```python
from build123d import *

# Parameters (mm, degrees)
SKETCH1_W           = 28.7
SKETCH1_H           = 30.1
BOSS_EXTRUDE1_DEPTH = 10.3
SKETCH2_W           = 22
SKETCH2_H           = 20.1
SKETCH2_R           = 0.95
BOSS_EXTRUDE2_DEPTH = 4
SKETCH4_R           = 0.95
CUT_EXTRUDE1_DEPTH  = 44.979427009


with BuildPart() as part:
    # Sketch1 → Boss-Extrude1 (new body)
    with BuildSketch(Plane.XY):
        with Locations((14.35, 15.05)):
            Rectangle(SKETCH1_W, SKETCH1_H)
    extrude(amount=BOSS_EXTRUDE1_DEPTH)

    # Sketch2 → Boss-Extrude2 (add)
    with BuildSketch(Plane.XY.offset(10.3)):
        with Locations((14.35, 15.05)):
            Rectangle(SKETCH2_W, SKETCH2_H)
        with Locations((6.967324962, 8.304919624)):
            Circle(SKETCH2_R, mode=Mode.SUBTRACT)
        with Locations(Location((6.967324962, 21.795080376, 0), (0, 0, 180))):
            Circle(SKETCH2_R, mode=Mode.SUBTRACT)
        with Locations(Location((21.732675038, 8.304919624, 0), (0, 0, 180))):
            Circle(SKETCH2_R, mode=Mode.SUBTRACT)
        with Locations((21.732675038, 21.795080376)):
            Circle(SKETCH2_R, mode=Mode.SUBTRACT)
    extrude(amount=BOSS_EXTRUDE2_DEPTH)

    # Sketch4 → Cut-Extrude1 (cut, through all)
    with BuildSketch(Plane(origin=(0, 0, 0), x_dir=(-1, 0, 0), z_dir=(0, 0, -1))):
        with Locations((-21.732675038, 21.795080376)):
            Circle(SKETCH4_R)
        with Locations((-21.732675038, 8.304919624)):
            Circle(SKETCH4_R)
        with Locations((-6.967324962, 8.304919624)):
            Circle(SKETCH4_R)
        with Locations((-6.967324962, 21.795080376)):
            Circle(SKETCH4_R)
    extrude(amount=-CUT_EXTRUDE1_DEPTH, mode=Mode.SUBTRACT)


solid = part.part
```
Could you check a few things on this model? Use its own coordinates, in mm. A direction names the side the tool comes from. Round coordinates to 2 decimals unless told otherwise and drop trailing zeros. Loops run counter-clockwise (first coordinate to the right, second up) from the corner with the lowest first, then second, coordinate; pieces in that order, holes last. Notation, with made-up numbers: M 89.25,12.25 L 127.25,12.25 A11 cw 127.25,30.25 Z; hole C 35,26 d1. An arc over 180 degrees is marked long. Put each result on its own line as item: value.
Q1. Thinking about a two-plate mould opening in Y: for faces 1 (the face through (28.7, 15, 5)), 2 (the face through (20.827, 8.59, 7.05)), 3 (the face through (14, 5, 12)), which applies, released by +Y, released by -Y, zero draft, split by the parting line, or undercut?
Check result:
face 1: zero draft
face 2: undercut
face 3: released by -Y
Q2. For pin 1 (5 mm diameter, centred on x = 24, z = 1.5, fed in from -Y); pin 2 (3 mm diameter, centred on x = 17.5, z = 12, fed in from +Y); pin 3 (3 mm diameter, centred on y = 19.5, z = 12.5, fed in from -X); pin 4 (3 mm diameter, centred on x = 10, z = 12.5, fed in from -Y), each with a flat end and sliding along its axis, tell me the tip position at first contact or that it passes through.
Check result:
pin 1: y = 0
pin 2: y = 25.1
pin 3: x = 3.35
pin 4: y = 5
Q3. Imagine slicing it at A-A (x = 4). Write out the boundary of the cut face in (y, z).
Check result:
outline: M 0,0 L 30.1,0 L 30.1,10.3 L 25.1,10.3 L 25.1,14.3 L 5,14.3 L 5,10.3 L 0,10.3 Z
Q4. I need wall thicknesses on probe 1 along X at (y, z) = (21, 9.25); probe 2 along X at (y, z) = (22, 9.5); probe 3 along Y at (x, z) = (18.5, 10.75). Which ranges of each line are inside material? Lowest first, please.
Check result:
probe 1: 0 to 6.45, 7.49 to 21.21, 22.25 to 28.7
probe 2: 0 to 6.04, 7.89 to 20.81, 22.66 to 28.7
probe 3: 5 to 25.1
Q5. Imagine slicing it at C-C (y = 13.5). Write out the boundary of the cut face in (x, z).
Check result:
outline: M 0,0 L 28.7,0 L 28.7,10.3 L 25.35,10.3 L 25.35,14.3 L 3.35,14.3 L 3.35,10.3 L 0,10.3 Z
Q6. On a 3-axis mill with a long thin cutter (end or side, diameter ignored), from which of +Z, -Z, +X, -X, +Y, -Y can I reach the whole of each face in a straight line? I mean faces 4 (the face through (14, 25.1, 12)), 5 (the face through (3.35, 15, 12)), 6 (the face through (25.35, 15, 12)). Say none if no direction works.
Check result:
face 4: +Z, +X, -X, +Y
face 5: +Z, -X, +Y, -Y
face 6: +Z, +X, +Y, -Y
Q7. Imagine slicing it at B-B (z = 10.75). Write out the boundary of the cut face in (x, y).
Check result:
outline: M 3.35,5 L 25.35,5 L 25.35,25.1 L 3.35,25.1 Z; hole C 6.97,8.3 d1.9; hole C 6.97,21.8 d1.9; hole C 21.73,8.3 d1.9; hole C 21.73,21.8 d1.9
Q8. Imagine slicing it at D-D (y = 27.5). Write out the boundary of the cut face in (x, z), then the cut area to 3 significant figures.
Check result:
outline: M 0,0 L 28.7,0 L 28.7,10.3 L 0,10.3 Z
area: 296 mm2
